Read the model definition and answer for the solid it produces. Units are mm, in the model's axes. A direction names the side the tool comes from. Coordinates: 2 decimals unless noted, no trailing zeros. Loops run counter-clockwise (first coordinate to the right, second up) from the corner with the lowest first, then second, coordinate; pieces in that order, holes last.
Q1. Flat-ended cylindrical pins translate along their axes: P1, Ø2, axis at x = 0, z = 5.5, coming from the -Y side; P2, Ø4, axis at x = 5, z = 0, coming from the +Y side; P3, Ø4, axis at x = -5, z = 4.5, coming from the +Y side. Find the tip coordinate at first contact, or state that the pin passes through.
Q2. Section A-A (y = 1.25) is taken. Give the vertices of the cut face in (x, z) (3 decimals), then the cut area to 3 significant figures.
Q3. Section B-B (z = -2.5) is taken. Give the vertices of the cut face in (x, y).
Q4. Straight lines are drawn through the part: line 1 (X direction, y = 1, z = 0); line 2 (Z direction, x = 3.5, y = 1) (3 decimals); line 3 (Y direction, x = -0.5, z = 0.5). For each, find the intervals that lie inside material, in ascending order.
Q5. Which of the six approach directions +Z, -Z, +X, -X, +Y, -Y give full straight-line access (tool end or side, diameter ignored) to faces 5 (the face through (-6.43, 4.09, 0.39)), 6 (the face through (0.45, 1.01, -1.43)), 7 (the face through (0.022, -0.625, 7.405)), 8 (the face through (0, 0, 3))?
Q6. Section C-C (z = 6.75) is taken. Give the vertices of the cut face in (x, y).
Q7. The mould has two halves that part along X. Classify faces 1 (the face through (1.6, 2, 6)), 2 (the face through (0, 2, 0)), 3 (the face through (-1.6, 2, 6)), 4 (the face through (-5, 2, 3.975)): pulls with the +X half, pulls with the -X half, needs draft (parallel to the pull), parting line crosses it, or undercut.
Q8. Section D-D (x = 3.95) is taken. Give the vertices of the cut face in (y, z) (3 decimals).
from build123d import *

# Parameters (mm, degrees)
SKETCH1_W           = 15.9
SKETCH1_H           = 7.95
BOSS_EXTRUDE1_DEPTH = 3.2
SHELL1_T            = -1.2
SKETCH3_R           = 1.5
SKETCH3_R_2         = 0.5
BOSS_EXTRUDE3_DEPTH = 2
SKETCH4_R           = 2.4
BOSS_EXTRUDE4_DEPTH = 1.8
LPATTERN1_COUNT     = 2
LPATTERN1_PITCH     = 8
BOSS_EXTRUDE5_DEPTH = 1.6


with BuildPart() as part:
    # Sketch1 → Boss-Extrude1 (new body)
    with BuildSketch(Plane(origin=(0, 0, 0), x_dir=(1, 0, 0), z_dir=(0, 1, 0))):
        Rectangle(SKETCH1_W, SKETCH1_H)
    extrude(amount=BOSS_EXTRUDE1_DEPTH)

    # Shell1
    shell1_openings = [part.faces().sort_by_distance(p)[0] for p in [
        (0, 0, 0),
    ]]
    offset(amount=SHELL1_T, openings=shell1_openings, kind=Kind.INTERSECTION)

    # Sketch3 → Boss-Extrude3 (add)
    with BuildSketch(Plane.XZ.offset(-2)):
        with Locations(Location((0, 0, 0), (0, 0, 270))):
            Circle(SKETCH3_R)
        with Locations(Location((0, 0, 0), (0, 0, 270))):
            Circle(SKETCH3_R_2, mode=Mode.SUBTRACT)
    extrude(amount=BOSS_EXTRUDE3_DEPTH)

    # Sketch4 → Boss-Extrude4 (add)
    with BuildSketch(Plane(origin=(0, 3.2, 0), x_dir=(1, 0, 0), z_dir=(0, 1, 0))):
        with Locations(Location((-4.05, -0.075, 0), (0, 0, 90))):
            Circle(SKETCH4_R)
    boss_extrude4 = extrude(amount=BOSS_EXTRUDE4_DEPTH)

    # LPattern1: Boss-Extrude4 ×2
    with Locations(*[(i * LPATTERN1_PITCH, 0, 0) for i in range(1, LPATTERN1_COUNT)]):
        add(boss_extrude4)

    # Sketch5 → Boss-Extrude5 (add, symmetric)
    with BuildSketch(Plane(origin=(0, 0, 0), x_dir=(0, 0, -1), z_dir=(1, 0, 0))):
        with BuildLine():
            Line((-3.975, 0), (-5.975, 0))
            ThreePointArc((-5.975, 0), (-7.427655013, -0.628062458), (-8.997768861, -0.429539046))
            ThreePointArc((-8.997768861, -0.429539046), (-9.403665936, 0.550383177), (-8.423743712, 0.956280252))
            ThreePointArc((-8.423743712, 0.956280252), (-6.349718564, 2.342099551), (-8.423743712, 3.72791885))
            ThreePointArc((-8.423743712, 3.72791885), (-9.403665936, 4.133815925), (-8.997768861, 5.113738149))
            ThreePointArc((-8.997768861, 5.113738149), (-6.560942303, 5.051168718), (-4.975, 3.2))
            Line((-4.975, 3.2), (-3.975, 3.2))
            Line((-3.975, 3.2), (-3.975, 0))
        make_face()
    extrude(amount=BOSS_EXTRUDE5_DEPTH, both=True)


solid = part.part
Numbers:
1. P1: stops at y = -0.34
1. P2: stops at y = 5
1. P3: stops at y = 3.2
2. outline: (-7.95, -3.975) - (7.95, -3.975) - (7.95, 3.975) - (1.6, 3.975) - (1.6, 6.821) - (-1.6, 6.821) - (-1.6, 3.975) - (-7.95, 3.975) - close; circle Ø3 at (0, 0); hole (-6.75, -2.775) - (6.75, -2.775) - (6.75, 2.775) - (-6.75, 2.775) - close; hole circle Ø1 at (0, 0)
2. area: 66.9 mm2
3. outline: (-7.95, 0) - (-6.75, 0) - (-6.75, 2) - (6.75, 2) - (6.75, 0) - (7.95, 0) - (7.95, 3.2) - (-7.95, 3.2) - close
4. line 1: x = -7.95 to -6.75, -1.5 to -0.5, 0.5 to 1.5, 6.75 to 7.95
4. line 2: z = -3.975 to -2.775, 2.775 to 3.975
4. line 3: y = 0 to 3.2
5. face 5: +Y
5. face 6: -Y
5. face 7: +X, -X, -Y
5. face 8: -Z, +X, -X, -Y
6. outline: (-1.6, -0.45) - (1.6, -0.45) - (1.6, 1.32) - (-1.6, 1.32) - close; (-1.6, 3.36) - (1.6, 3.36) - (1.6, 5.13) - (-1.6, 5.13) - close
7. face 1: pulls with the +X half
7. face 2: undercut
7. face 3: pulls with the -X half
7. face 4: needs draft
8. outline: (0, -3.975) - (3.2, -3.975) - (3.2, -2.325) - (5, -2.325) - (5, 2.475) - (3.2, 2.475) - (3.2, 3.975) - (0, 3.975) - (0, 2.775) - (2, 2.775) - (2, -2.775) - (0, -2.775) - close
